from build123d import *

# Parameters (mm, degrees)
F1_DEPTH = 9.525
F2_DEPTH = 9.525
F4_D     = 10.31875


# Not quite as in the source:
# - a feature of the source that left no trace in its solid (it failed there, or was rolled back) is left out


with BuildPart() as f1:
    # F0 (on Top) → F1 (new body)
    with BuildSketch(Plane.XY):
        Polygon((-266.7, -139.7), (101.6, -139.7), (101.6, -76.2), (101.6, 76.2), (101.6, 139.7), (-266.7, 139.7), align=None)
    extrude(amount=F1_DEPTH)

    # F0 (on Top) → F2 (join)
    with BuildSketch(Plane.XY):
        with BuildLine():
            Line((101.6, 76.2), (101.6, -76.2))
            ThreePointArc((101.6, -76.2), (112.7592316368, -49.2592316368), (139.7, -38.1))
            Line((139.7, -38.1), (228.6, -38.1))
            ThreePointArc((228.6, -38.1), (266.7, 0), (228.6, 38.1))
            Line((228.6, 38.1), (139.7, 38.1))
            ThreePointArc((139.7, 38.1), (112.7592316368, 49.2592316368), (101.6, 76.2))
        make_face()
        with BuildLine():
            Line((212.725, 9.525), (241.3, 9.525))
            ThreePointArc((241.3, 9.525), (250.825, 0), (241.3, -9.525))
            Line((241.3, -9.525), (212.725, -9.525))
            ThreePointArc((212.725, -9.525), (203.2, 0), (212.725, 9.525))
        make_face(mode=Mode.SUBTRACT)
    extrude(amount=F2_DEPTH)

    # F4 (through all)
    with Locations(Plane(origin=(0, 0, 0), x_dir=(1, 0, 0), z_dir=(0, 0, -1))):
        with Locations((-165.1, -88.9), (-165.1, 88.9), (50.8, 88.9), (50.8, -88.9)):
            Hole(F4_D / 2)


solid = f1.part
Geometry check sheet. Reference: the model listing, model coordinates, mm. A direction names the side the tool comes from. Coordinates: 2 decimals unless noted, no trailing zeros. Order: outer loops, then holes, each group sorted by start corner. A loop starts at its lowest first (then second) coordinate and runs counter-clockwise, first axis right, second up. Notation, with made-up numbers: (75.25, 76.25) - (93.25, 76.25) arc R26 ccw to (93.25, 111.25) - close; hole circle Ø10 at (-13, 39.25). An arc over 180 degrees is marked (long way). One line per item, written item: value.
(1) Sectioned sample at D-D (y = 0). Enter the section's corners in (x, z) (3 decimals).
Data:
outline: (-266.7, 0) - (203.2, 0) - (203.2, 9.525) - (-266.7, 9.525) - close; (250.825, 0) - (266.7, 0) - (266.7, 9.525) - (250.825, 9.525) - close
(2) Depth check by flat-ended pin: pin 1 Ø3 at (x, z) = (225.5, 4) entering from +Y; pin 2 Ø5 at (y, z) = (93.5, 6.5) entering from +X; pin 3 Ø5 at (x, z) = (225.5, 7) entering from -Y; pin 4 Ø8.5 at (x, y) = (50.8, -88.9) entering from -Z. Enter the tip coordinate at first touch or a pass-through.
Data:
pin 1: stops at y = 38.1
pin 2: stops at x = 101.6
pin 3: stops at y = -38.1
pin 4: passes through
(3) Sectioned sample at B-B (z = 1.5). Enter the section's corners in (x, y) (3 decimals).
Data:
outline: (-266.7, -139.7) - (101.6, -139.7) - (101.6, -76.2) arc R38.1 cw to (139.7, -38.1) - (228.6, -38.1) arc R38.1 ccw to (228.6, 38.1) - (139.7, 38.1) arc R38.1 cw to (101.6, 76.2) - (101.6, 139.7) - (-266.7, 139.7) - close; hole circle Ø10.319 at (-165.1, -88.9); hole circle Ø10.319 at (-165.1, 88.9); hole circle Ø10.319 at (50.8, -88.9); hole circle Ø10.319 at (50.8, 88.9); hole (212.725, -9.525) - (241.3, -9.525) arc R9.525 ccw to (241.3, 9.525) - (212.725, 9.525) arc R9.525 ccw to start
(4) Thickness scan on probe 1 along X at (y, z) = (88.9, 3.5); probe 2 along X at (y, z) = (90, 9); probe 3 along Y at (x, z) = (50.8, 3.5). Record the ranges inside material, lowest first. Write a range as from..to.
Data:
probe 1: x = -266.7..-170.26, -159.94..45.64, 55.96..101.6
probe 2: x = -266.7..-170.14, -160.06..45.76, 55.84..101.6
probe 3: y = -139.7..-94.06, -83.74..83.74, 94.06..139.7
(5) Sectioned sample at C-C (x = 50.8). Enter the section's corners in (y, z) (3 decimals).
Data:
outline: (-139.7, 0) - (-94.059, 0) - (-94.059, 9.525) - (-139.7, 9.525) - close; (-83.741, 0) - (83.741, 0) - (83.741, 9.525) - (-83.741, 9.525) - close; (94.059, 0) - (139.7, 0) - (139.7, 9.525) - (94.059, 9.525) - close
(6) Sectioned sample at A-A (y = 88.9). Enter the section's corners in (x, z) (3 decimals), and give its area (3 significant figures).
Data:
outline: (-266.7, 0) - (-170.259, 0) - (-170.259, 9.525) - (-266.7, 9.525) - close; (-159.941, 0) - (45.641, 0) - (45.641, 9.525) - (-159.941, 9.525) - close; (55.959, 0) - (101.6, 0) - (101.6, 9.525) - (55.959, 9.525) - close
area: 3,310 mm^2
(7) Access from +Z, -Z, +X, -X, +Y, -Y to the whole of each face (thin tool, end or side, straight path). Record for faces 5 (the face through (101.6, -108, 5)), 6 (the face through (266.69, -0.84, 4.7)), 7 (the face through (185, 38.1, 5)), 8 (the face through (-63, 2, 9.525)), 9 (the face through (227, -9.525, 5)).
Data:
face 5: +Z, -Z, +X, -Y
face 6: +Z, -Z, +X
face 7: +Z, -Z, +X, +Y
face 8: +Z, +X, -X, +Y, -Y
face 9: +Z, -Z
(8) Release check for a two-part mould opening along X. For faces 1 (the face through (-266.7, 2, 5)), 2 (the face through (184, -38.1, 5)), 3 (the face through (101.6, 108, 5)), 4 (the face through (227, 9.525, 5)) record: +X half, -X half, draft (parallel to the pull), parting line (faces both ways), or undercut.
Data:
face 1: -X half
face 2: draft
face 3: +X half
face 4: undercut
